from build123d import *

# Parameters (mm, degrees)
SKETCH_2_R        = 1.5
EXTRUDE_1_DEPTH   = 2
SKETCH_2_3_R      = 3
SKETCH_2_3_R_2    = 1.5
EXTRUDE_1_2_DEPTH = 5


with BuildPart() as part:
    # 草图2 → Extrude 1 (new body)
    with BuildSketch(Plane(origin=(0, 0, 0), x_dir=(1, 0, 0), z_dir=(0, 1, 0))):
        with BuildLine():
            ThreePointArc((-16.914467174, 6.15636258), (-17.726539554, 3.125667198), (-18, 0))
            ThreePointArc((-18, 0), (-14.5, -3.5), (-11, 0))
            ThreePointArc((-11, 0), (-10.832885283, 1.910129954), (-10.336618829, 3.762221577))
            ThreePointArc((-10.336618829, 3.762221577), (-12.4284725, 8.248216251), (-16.914467174, 6.15636258))
        make_face()
        with Locations(Location((-14.279712419, 2.517898576, 0), (0, 0, 270))):
            Circle(SKETCH_2_R, mode=Mode.SUBTRACT)
    extrude(amount=EXTRUDE_1_DEPTH)

    # 草图2<3> → Extrude 1 2 (add)
    with BuildSketch(Plane(origin=(0, 0, 0), x_dir=(1, 0, 0), z_dir=(0, 1, 0))):
        with Locations((-14.279712419, 2.517898576)):
            Circle(SKETCH_2_3_R)
        with Locations((-14.279712419, 2.517898576)):
            Circle(SKETCH_2_3_R_2, mode=Mode.SUBTRACT)
    extrude(amount=EXTRUDE_1_2_DEPTH)


solid = part.part
Geometry: final body of the model. Coordinates: model frame, mm. A direction names the side the tool comes from. Give positions to 0.01 mm unless a question says otherwise; leave off trailing zeros. Loops run counter-clockwise (first coordinate to the right, second up) from the corner with the lowest first, then second, coordinate; pieces in that order, holes last. Notation, with made-up numbers: (-33.5, 84) -> (3.5, 84) arc R28 ccw to (3.5, 104) -> close; hole circle Ø1 at (-26, 12.25). An arc over 180 degrees is marked (long way). Put each result on its own line as item: value.
1. Pin query (flat end, axial travel): P1, Ø1, axis at y = 2, z = -3, coming from the -X side; P2, Ø2, axis at x = -16, y = 3.5, coming from the -Z side. Return the tip coordinate at first contact, or that it passes through.
Taken from the geometry:
P1: stops at x = -17.83
P2: stops at z = -5.43
2. Ray query, line 1 along Z through (x, y) = (-14.25, 3.95); line 2 along Y through (x, z) = (-12.75, 1.25); line 3 along Z through (x, y) = (-13.5, 2.1). Return the intervals inside material, ascending. Write a range as [from, to].
Taken from the geometry:
line 1: z = [-5.52, -4.02], [-1.02, 0.48]
line 2: y = [0, 2]
line 3: z = [-5.41, -3.8], [-1.24, 0.38]
3. Cut plane C-C (x = -12). Return the cut outline in (y, z), plus the area to 3 significant figures.
Taken from the geometry:
outline: (0, -8.06) -> (2, -8.06) -> (2, -4.47) -> (5, -4.47) -> (5, -0.57) -> (2, -0.57) -> (2, 2.45) -> (0, 2.45) -> close
area: 32.7 mm2
4. Cut plane A-A (x = -14.5). Return the cut outline in (y, z).
Taken from the geometry:
outline: (0, -8.35) -> (2, -8.35) -> (2, -5.51) -> (5, -5.51) -> (5, -4) -> (0, -4) -> close; (0, -1.03) -> (5, -1.03) -> (5, 0.47) -> (2, 0.47) -> (2, 3.5) -> (0, 3.5) -> close
5. Pull-direction query (Z, two-part tool) for faces 3 (the cylindrical face through (-13.721, 1.909, -1.126)), 4 (the flat face through (-13, 0, -1)), 5 (the cylindrical face through (-17.72, 0.99, -3.17)), 6 (the cylindrical face through (-14.6, 1, 3.5)); classes: released by +Z, released by -Z, zero draft, split by the parting line, or undercut.
Taken from the geometry:
face 3: undercut
face 4: zero draft
face 5: released by -Z
face 6: released by +Z
6. Set-up query: faces 1 (the flat face through (-16, 5, -2)), 2 (the cylindrical face through (-17.277, 3.479, -2.65)). Return all of +Z, -Z, +X, -X, +Y, -Y with unobstructed straight access to the full face (end or side cutting, diameter ignored); none if empty.
Taken from the geometry:
face 1: +Z, -Z, +X, -X, +Y
face 2: +Y
7. Cut plane D-D (z = -7.5). Return the cut outline in (x, y), plus the area to 3 significant figures.
Taken from the geometry:
outline: (-16.03, 0) -> (-11.22, 0) -> (-11.22, 2) -> (-16.03, 2) -> close
area: 9.63 mm2
